from build123d import *

# Parameters (mm, degrees)
SKETCH_1_W          = 160
SKETCH_1_H          = 180
EXTRUDE_1_DEPTH     = 4
SKETCH_2_W          = 150
SKETCH_2_H          = 175
CUT_EXTRUDE_1_DEPTH = 1
SKETCH_3_R          = 2.5
EXTRUDE_2_DEPTH     = 10


with BuildPart() as part:
    # 草图1 → 凸台-拉伸1 (new, symmetric)
    with BuildSketch(Plane.XY):
        Rectangle(SKETCH_1_W, SKETCH_1_H)
    extrude(amount=EXTRUDE_1_DEPTH, both=True)

    # 草图2 → 切除-拉伸1 (cut)
    with BuildSketch(Plane.XY.offset(4)):
        with Locations((0, -2.5)):
            Rectangle(SKETCH_2_W, SKETCH_2_H)
    extrude(amount=-CUT_EXTRUDE_1_DEPTH, mode=Mode.SUBTRACT)

    # 草图3 → 凸台-拉伸2 (add, symmetric)
    with BuildSketch(Plane.XY):
        with Locations(Location((-77.5, -80, 0), (0, 0, 180))):
            Circle(SKETCH_3_R)
        with Locations(Location((77.5, -80, 0), (0, 0, 180))):
            Circle(SKETCH_3_R)
    extrude(amount=EXTRUDE_2_DEPTH, both=True)


solid = part.part
Here's how the part is built. I have some questions about the finished solid (model axes, mm). A direction names the side the tool comes from. Round coordinates to 2 decimals unless told otherwise and drop trailing zeros. Loops run counter-clockwise (first coordinate to the right, second up) from the corner with the lowest first, then second, coordinate; pieces in that order, holes last. Notation, with made-up numbers: M -3,-33 L 1,-33 A18 cw 1,-25 Z; hole C -32,33.5 d11. An arc over 180 degrees is marked long. Write each question's results on one line, items separated by ' | '. Start each with the question number.
(1) On a 3-axis mill with a long thin cutter (end or side, diameter ignored), from which of +Z, -Z, +X, -X, +Y, -Y can I reach the whole of each face in a straight line? I mean faces 1 (the cylindrical face through (-75, -80, 7)), 2 (the cylindrical face through (-75, -80, -7)), 3 (the flat face through (-1, 90, 0)), 4 (the flat face through (-1, -1, 3)), 5 (the flat face through (78, -80, -10)). Say none if no direction works.
(2) Thinking about a two-plate mould opening in X: for faces 6 (the flat face through (-77, -80, 10)), 7 (the flat face through (80, -1, 0)), 8 (the cylindrical face through (80, -80, 7)), which applies, pulls with the +X half, pulls with the -X half, needs draft (parallel to the pull), parting line crosses it, or undercut?
(3) I want a section at A-A (z = -6). Please give me the cut outline in (x, y), then the cut area to 3 significant figures.
(4) I want a section at B-B (x = 77.5). Please give me the cut outline in (y, z).
(5) Will these pins go through, and if not, where does the flat tip stop? P1, Ø5, axis at x = -56.5, y = 7.5, coming from the -Z side; P2, Ø0.8, axis at x = -2.5, z = 3.5, coming from the -Y side; P3, Ø1.5, axis at x = 77.5, y = -84, coming from the +Z side.
(6) I want a section at D-D (x = -36.5). Please give me the cut outline in (y, z), then the cut area to 4 significant figures.
(7) If I drill on probe 1 along Z at (x, y) = (32.5, -23), over which ranges is the centre line in solid material (lowest first)? Write a range as from..to.
(8) I want a section at C-C (y = 35.5). Please give me the cut outline in (x, z).
Solved:
1) face 1: +Z | face 2: -Z | face 3: +Z, -Z, +X, -X, +Y | face 4: +Z, -Y | face 5: -Z, +X, -X, +Y, -Y
2) face 6: needs draft | face 7: pulls with the +X half | face 8: undercut
3) outline: C -77.5,-80 d5; C 77.5,-80 d5 | area: 39.3 mm²
4) outline: M -90,-4 L -82.5,-4 L -82.5,-10 L -77.5,-10 L -77.5,-4 L 90,-4 L 90,4 L -77.5,4 L -77.5,10 L -82.5,10 L -82.5,4 L -90,4 Z
5) P1: stops at z = -4 | P2: stops at y = 85 | P3: stops at z = 4
6) outline: M -90,-4 L 90,-4 L 90,4 L 85,4 L 85,3 L -90,3 Z | area: 1,265 mm²
7) probe 1: z = -4..3
8) outline: M -80,-4 L 80,-4 L 80,4 L 75,4 L 75,3 L -75,3 L -75,4 L -80,4 Z
